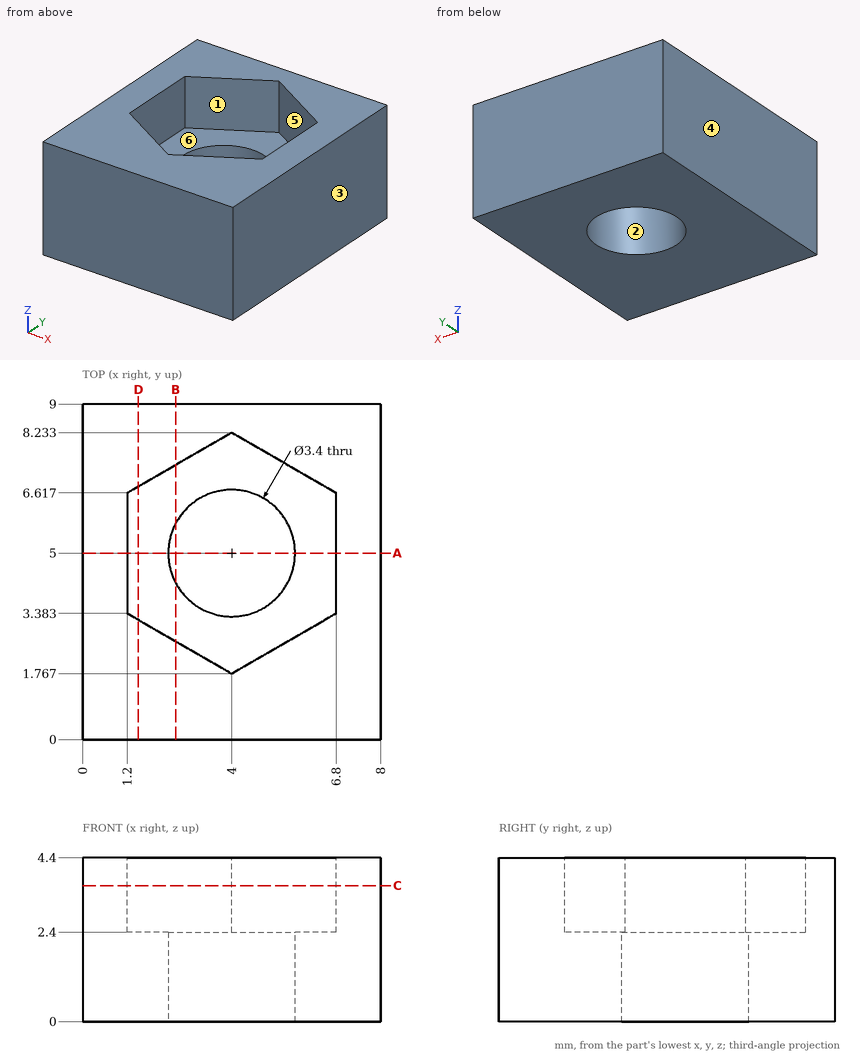
Verification items for this drawing (mm, ordinates from the low corner). A direction names the side the tool comes from. Round coordinates to 2 decimals unless told otherwise and drop trailing zeros. Order: outer loops, then holes, each group sorted by start corner. A loop starts at its lowest first (then second) coordinate and runs counter-clockwise, first axis right, second up. Notation, with made-up numbers: M 8,-38 L 14,-38 A8 cw 14,-33 Z; hole C 64,82.5 d1. An arc over 180 degrees is marked long. Answer in a Markdown table with one row per item. Add a question column.
Item 1: Sectioned sample at C-C, the plane z = 3.65. Enter the section's corners in (x, y).
Item 2: Set-up check for the marked faces 1 and 2: record each of +Z, -Z, +X, -X, +Y, -Y from which the full face is reachable in a straight line by a thin tool's end or side.
Item 3: Sectioned sample at D-D, the plane x = 1.5. Enter the section's corners in (y, z).
Item 4: Draft check along X on the marked faces 3, 4, 5 and 6. Enter one of: released by +X, released by -X, zero draft, split by the parting line, or undercut.
Item 5: Material ranges on L1, parallel to Y at x = 4, z = 0.9; L2, parallel to X at y = 5, z = 0.7; L3, parallel to X at y = 6.5, z = 2.8, recorded low to high. Write a range as [from, to].
Item 6: Sectioned sample at A-A, the plane y = 5. Enter the section's corners in (x, z).
Item 7: Depth check by flat-ended pin: pin 1 Ø1.7 at (x, y) = (4.5, 6) entering from +Z. Enter the tip coordinate at first touch or a pass-through.
Item 8: Sectioned sample at B-B, the plane x = 2.5. Enter the section's corners in (y, z), plus the area to 3 significant figures.
Filled in:
| question | item | result |
|---|---|---|
| 1 | outline | M 0,0 L 8,0 L 8,9 L 0,9 Z; hole M 1.2,3.38 L 4,1.77 L 6.8,3.38 L 6.8,6.62 L 4,8.23 L 1.2,6.62 Z |
| 2 | face 1 | +Z |
| 2 | face 2 | +Z, -Z |
| 3 | outline | M 0,0 L 9,0 L 9,4.4 L 6.79,4.4 L 6.79,2.4 L 3.21,2.4 L 3.21,4.4 L 0,4.4 Z |
| 4 | face 3 | released by +X |
| 4 | face 4 | released by -X |
| 4 | face 5 | undercut |
| 4 | face 6 | undercut |
| 5 | L1 | y = [0, 3.3], [6.7, 9] |
| 5 | L2 | x = [0, 2.3], [5.7, 8] |
| 5 | L3 | x = [0, 1.2], [6.8, 8] |
| 6 | outline | M 0,0 L 2.3,0 L 2.3,2.4 L 1.2,2.4 L 1.2,4.4 L 0,4.4 Z; M 5.7,0 L 8,0 L 8,4.4 L 6.8,4.4 L 6.8,2.4 L 5.7,2.4 Z |
| 7 | pin 1 | stops at z = 2.4 |
| 8 | outline | M 0,0 L 4.2,0 L 4.2,2.4 L 2.63,2.4 L 2.63,4.4 L 0,4.4 Z; M 5.8,0 L 9,0 L 9,4.4 L 7.37,4.4 L 7.37,2.4 L 5.8,2.4 Z |
| 8 | area | 26.3 mm² |
